from build123d import *

# Parameters (mm, degrees)
BOSS_EXTRUDE1_DEPTH                            = 12.7
SKETCH2_W                                      = 25.4
SKETCH2_H                                      = 19.05
BOSS_EXTRUDE2_DEPTH                            = 3.175
FILLET1_R                                      = 3.175
F_17_64_0_26563_DIAMETER_HOLE1_D               = 6.747002
CSK_FOR_6_FLAT_HEAD_MACHINE_SCREW1_D           = 3.7973
CSK_FOR_6_FLAT_HEAD_MACHINE_SCREW1_DEPTH       = 16.51
CSK_FOR_6_FLAT_HEAD_MACHINE_SCREW1_CSINK_D     = 7.0866
CSK_FOR_6_FLAT_HEAD_MACHINE_SCREW1_CSINK_ANGLE = 82
CSK_FOR_6_FLAT_HEAD_MACHINE_SCREW1_TIP         = 1.140824014
CSK_FOR_6_FLAT_HEAD_MACHINE_SCREW2_D           = 3.7973
CSK_FOR_6_FLAT_HEAD_MACHINE_SCREW2_DEPTH       = 16.51
CSK_FOR_6_FLAT_HEAD_MACHINE_SCREW2_CSINK_D     = 7.0866
CSK_FOR_6_FLAT_HEAD_MACHINE_SCREW2_CSINK_ANGLE = 82
CSK_FOR_6_FLAT_HEAD_MACHINE_SCREW2_TIP         = 1.140824014


with BuildPart() as part:
    # Sketch1 → Boss-Extrude1 (new body)
    with BuildSketch(Plane(origin=(0, 0, 0), x_dir=(1, 0, 0), z_dir=(0, 1, 0))):
        Polygon((0, 15.875), (0, -15.875), (34.925, -15.875), (34.925, -9.525), (9.525, -9.525), (9.525, 9.525), (34.925, 9.525), (34.925, 15.875), align=None)
    extrude(amount=BOSS_EXTRUDE1_DEPTH)

    # Sketch2 → Boss-Extrude2 (add)
    with BuildSketch(Plane.XZ):
        with Locations((22.225, 0)):
            Rectangle(SKETCH2_W, SKETCH2_H)
    extrude(amount=-BOSS_EXTRUDE2_DEPTH)

    # Fillet1
    fillet1_edges = [part.edges().sort_by_distance(p)[0] for p in [
        (9.525, 7.9375, -9.525),
        (9.525, 7.9375, 9.525),
    ]]
    fillet(fillet1_edges, radius=FILLET1_R)

    # 17/64 (0.26563) Diameter Hole1 (through all)
    with Locations(Plane.ZY):
        with Locations((0, 7.9375)):
            Hole(F_17_64_0_26563_DIAMETER_HOLE1_D / 2)

    # CSK for #6 Flat Head Machine Screw1
    with Locations(Plane(origin=(0, 12.7, 0), x_dir=(1, 0, 0), z_dir=(0, 1, 0))):
        with Locations((4.7625, -11.1125), (4.7625, 11.1125)):
            CounterSinkHole(CSK_FOR_6_FLAT_HEAD_MACHINE_SCREW1_D / 2, CSK_FOR_6_FLAT_HEAD_MACHINE_SCREW1_CSINK_D / 2, depth=CSK_FOR_6_FLAT_HEAD_MACHINE_SCREW1_DEPTH, counter_sink_angle=CSK_FOR_6_FLAT_HEAD_MACHINE_SCREW1_CSINK_ANGLE)
            with Locations((0, 0, -(CSK_FOR_6_FLAT_HEAD_MACHINE_SCREW1_DEPTH + CSK_FOR_6_FLAT_HEAD_MACHINE_SCREW1_TIP / 2))):  # 118° drill point
                Cone(0, CSK_FOR_6_FLAT_HEAD_MACHINE_SCREW1_D / 2, CSK_FOR_6_FLAT_HEAD_MACHINE_SCREW1_TIP, mode=Mode.SUBTRACT)

    # CSK for #6 Flat Head Machine Screw2
    with Locations(Plane(origin=(0, 3.175, 0), x_dir=(1, 0, 0), z_dir=(0, 1, 0))):
        with Locations((28.575, 0)):
            CounterSinkHole(CSK_FOR_6_FLAT_HEAD_MACHINE_SCREW2_D / 2, CSK_FOR_6_FLAT_HEAD_MACHINE_SCREW2_CSINK_D / 2, depth=CSK_FOR_6_FLAT_HEAD_MACHINE_SCREW2_DEPTH, counter_sink_angle=CSK_FOR_6_FLAT_HEAD_MACHINE_SCREW2_CSINK_ANGLE)
            with Locations((0, 0, -(CSK_FOR_6_FLAT_HEAD_MACHINE_SCREW2_DEPTH + CSK_FOR_6_FLAT_HEAD_MACHINE_SCREW2_TIP / 2))):  # 118° drill point
                Cone(0, CSK_FOR_6_FLAT_HEAD_MACHINE_SCREW2_D / 2, CSK_FOR_6_FLAT_HEAD_MACHINE_SCREW2_TIP, mode=Mode.SUBTRACT)


solid = part.part
Input: part model. Units: mm. Frame: model coordinates. A direction names the side the tool comes from. Round coordinates to 2 decimals unless told otherwise and drop trailing zeros. Order: outer loops, then holes, each group sorted by start corner. A loop starts at its lowest first (then second) coordinate and runs counter-clockwise, first axis right, second up. Notation, with made-up numbers: (76.25, 78.5) - (116.25, 78.5) arc R17 ccw to (116.25, 82.5) - close; hole circle Ø8 at (4.5, 80.25). An arc over 180 degrees is marked (long way). Answer as a JSON object with one key per item and string values. Group by question number.
(1) Cut plane C-C (x = 17.5). Return loops of the section in (y, z) (3 decimals).
(2) Cut plane B-B (y = 8.5). Count the separate pieces of the cut face and the enclosed holes in it, then the cut area to 3 significant figures.
(3) Cut plane D-D (z = 4.5). Return loops of the section in (x, y) (3 decimals).
(4) Reachability of faces 5 (the face through (17, 6, 15.875)), 6 (the face through (10.43, 8, -8.57)) from +Z, -Z, +X, -X, +Y, -Y: full face, straight path, thin tool, end or side. Return the list, or none.
(5) Material intervals for probe 1 along Y at (x, z) = (5.5, 0); probe 2 along Z at (x, y) = (6.5, 12) (3 decimals); probe 3 along Z at (x, y) = (6, 8.75) (3 decimals), sorted ascending. Write a range as from..to.
(6) Draft query along Y for faces 1 (the face through (17, 0, 0)), 2 (the face through (4.829, 11.282, 0.439)), 3 (the face through (10.48, 8, 8.62)), 4 (the face through (27.7, 1.4, 1.8)). Return one class per face: released by +Y, released by -Y, zero draft, split by the parting line, or undercut.
(7) Cut plane A-A (z = 0). Return loops of the section in (x, y) (3 decimals), then the cut area to 3 significant figures.
(8) Pin query (flat end, axial travel): P1, Ø15, axis at x = 21, z = -4.5, coming from the +Y side; P2, Ø1.5, axis at x = 16.5, z = 7, coming from the +Y side (3 decimals); P3, Ø4.5, axis at x = 4.76, z = 11.11, coming from the +Y side; P4, Ø1, axis at y = 7, z = 3, coming from the +X side (3 decimals). Return the tip coordinate at first contact, or that it passes through.
Here are the results:
{
 "1": {"outline": "(0, -15.875) - (12.7, -15.875) - (12.7, -9.525) - (3.175, -9.525) - (3.175, 9.525) - (12.7, 9.525) - (12.7, 15.875) - (0, 15.875) - close"},
 "2": {"separate pieces": "2", "enclosed holes": "2", "area": "543 mm^2"},
 "3": {"outline": "(0, 0) - (34.925, 0) - (34.925, 3.175) - (9.525, 3.175) - (9.525, 12.7) - (0, 12.7) - close"},
 "4": {"face 5": "+Z, +X, -X, +Y, -Y", "face 6": "+X, +Y"},
 "5": {"probe 1": "y = 0..4.56, 11.31..12.7", "probe 2": "z = -15.875..-13.478, -8.747..8.747, 13.478..15.875", "probe 3": "z = -15.875..-12.552, -9.673..-3.274, 3.274..9.673, 12.552..15.875"},
 "6": {"face 1": "released by -Y", "face 2": "undercut", "face 3": "zero draft", "face 4": "released by +Y"},
 "7": {"outline": "(0, 0) - (26.676, 0) - (26.676, 1.283) - (25.032, 3.175) - (9.525, 3.175) - (9.525, 4.564) - (0, 4.564) - close; (0, 11.311) - (9.525, 11.311) - (9.525, 12.7) - (0, 12.7) - close; (30.474, 0) - (34.925, 0) - (34.925, 3.175) - (32.118, 3.175) - (30.474, 1.283) - close", "area": "122 mm^2"},
 "8": {"P1": "stops at y = 12.7", "P2": "stops at y = 3.175", "P3": "stops at y = 11.22", "P4": "stops at x = 9.525"}
}
